Part model, mm, in its own coordinate system. A direction names the side the tool comes from. Give positions to 0.01 mm unless a question says otherwise; leave off trailing zeros. Write each loop counter-clockwise with the first axis right and the second up, starting at its lowest first coordinate (ties: lowest second). Pieces come first, ordered by that corner, then holes.
Autodesk Inventor part; units mm, degrees
ref_plane "YZ Plane" through (0, 0, 0) normal (1, 0, 0) x (0, 1, 0)
ref_plane "XZ Plane" through (0, 0, 0) normal (0, 1, 0) x (-1, 0, 0)
ref_plane "XY Plane" through (0, 0, 0) normal (0, 0, 1) x (1, 0, 0)
sketch "Sketch1" plane through (0, 0, 0) normal (0, 0, 1) x (1, 0, 0)
  line L0 (-25.4, 15.875) -> (-25.4, 3.175)
  line L1 (-25.4, 3.175) -> (9.525, 3.175)
  line L2 (9.525, 3.175) -> (9.525, 15.875)
  line L3 (9.525, 15.875) -> (-25.4, 15.875)
  dimension "d0" = 12.7
  dimension "d1" = 34.925
extrude "Extrusion1" add sketch "Sketch1" along normal blind 4.7625
hole "Hole1" at (3.175, 9.525, 4.7625) direction (0, 0, -1) diameter 4.318 end through all countersink diameter 8.4328 countersink angle 82
hole "Hole2" at (-9.525, 9.525, 4.7625) direction (0, 0, -1) diameter 3.302 end through all
sketch "Sketch2" plane through (0, 0, 4.7625) normal (0, 0, 1) x (1, 0, 0)
  line L0 (-25.4, 15.875) -> (9.525, 15.875)
  line L1 (-25.4, 3.175) -> (-25.4, 15.875)
  line L2 (-25.4, 11.1125) -> (-22.225, 11.1125)
  line L3 (-22.225, 11.1125) -> (-22.225, 7.9375)
  line L4 (-22.225, 7.9375) -> (-25.4, 7.9375)
  line L5 (-25.4, 7.9375) -> (-25.4, 11.1125)
  arc A0 (-22.225, 7.9375) -> (-22.225, 11.1125) centre (-22.225, 9.525) ccw
  dimension "d22" = 3.175
  dimension "d23" = 6.35
  dimension "d24" = 3.175
extrude "Extrusion2" cut sketch "Sketch2" against normal blind 1.016 contours L1 L2 L3 L4
sketch "Sketch6" plane through (-25.4, 3.175, 0) normal (0, -1, 0) x (1, 0, 0)
  line L0 (0, 0) -> (0, 4.7625)
  line L1 (0, 0) -> (34.925, 0)
  line L2 (0, 2.3813) -> (12.7, 0)
  line L3 (0, 0) -> (12.7, 0)
  line L4 (0, 0) -> (0, 2.3813)
  line L5 (0, 0) -> (12.7, 0)
  dimension "d35" = 2.3813
  dimension "d132" = 12.7
extrude "Extrusion5" cut sketch "Sketch6" against normal through all
hole "Hole4" at (-15.875, 13.4938, 4.7625) direction (0, 0, -1) diameter 0.7874 end through all
hole "Hole6" at (-15.875, 5.5563, 4.7625) direction (0, 0, -1) diameter 0.7874 end through all
sketch "Sketch8" plane through (0, 0, 4.7625) normal (0, 0, 1) x (1, 0, 0)
  line L0 (-25.4, 11.1125) -> (-22.225, 11.1125)
  line L1 (-22.225, 11.1125) -> (-22.225, 7.9375)
  line L2 (-25.4, 11.1125) -> (-22.225, 11.1125)
  line L3 (-22.225, 10.3187) -> (-25.4, 11.1125)
  line L4 (-22.225, 11.1125) -> (-22.225, 10.3187)
  line L5 (-22.225, 8.7312) -> (-25.4, 7.9375)
  line L6 (-22.225, 7.9375) -> (-22.225, 8.7312)
  dimension "d80" = 0.7937
  dimension "d81" = 0.7937
extrude "Extrusion7" add sketch "Sketch8" against normal up to next
sketch "Sketch10" plane through (0, 0, 4.7625) normal (0, 0, 1) x (1, 0, 0)
  line L0 (-22.225, 10.3187) -> (-22.225, 7.9375)
  line L1 (-22.225, 7.9375) -> (-25.4, 7.9375)
  line L2 (-22.225, 8.7312) -> (-25.4, 7.9375)
  line L3 (-22.225, 7.9375) -> (-22.225, 8.7312)
  dimension "d85" = 0.7937
extrude "Extrusion8" add sketch "Sketch10" against normal up to next
sketch "Sketch12" plane through (0, 0, 4.7625) normal (0, 0, 1) x (1, 0, 0)
  line L0 (-25.4, 15.875) -> (9.525, 15.875)
  line L1 (-25.4, 11.1125) -> (-25.4, 15.875)
  line L2 (-22.225, 10.3187) -> (-22.225, 8.7312)
  line L3 (-25.4, 11.9062) -> (-12.7, 15.875)
  line L4 (-25.4, 15.875) -> (-25.4, 11.9062)
  dimension "d88" = 12.7
  dimension "d89" = 3.9688
extrude "Extrusion9" cut sketch "Sketch12" against normal through all
sketch "Sketch13" plane through (0, 0, 4.7625) normal (0, 0, 1) x (1, 0, 0)
  line L0 (-25.4, 3.175) -> (-25.4, 7.9375)
  line L1 (9.525, 3.175) -> (-25.4, 3.175)
  line L2 (-12.7, 15.875) -> (9.525, 15.875)
  line L3 (-12.7, 3.175) -> (-25.4, 3.175)
  line L4 (-25.4, 7.1437) -> (-12.7, 3.175)
  dimension "d92" = 12.7
  dimension "d93" = 3.9688
extrude "Extrusion10" cut sketch "Sketch13" against normal through all
hole "Hole7" at (-0.7937, 13.4938, 4.7625) direction (0, 0, -1) diameter 2.159 end through all
hole "Hole8" at (-0.7937, 5.5562, 4.7625) direction (0, 0, -1) diameter 2.159 end through all
hole "Hole9" at (7.1437, 13.4938, 4.7625) direction (0, 0, -1) diameter 2.159 end through all
hole "Hole10" at (7.1437, 5.5562, 4.7625) direction (0, 0, -1) diameter 2.159 end through all
sketch "Sketch14" plane through (0, 0, 4.7625) normal (0, 0, 1) x (1, 0, 0)
  line L0 (-25.4, 11.1125) -> (-22.225, 10.3187)
  line L1 (-22.225, 8.7312) -> (-25.4, 7.9375)
  arc A0 (-22.225, 8.7312) -> (-22.225, 10.3187) centre (-22.4234, 9.525) ccw
  line L2 (-22.225, 10.3187) -> (-22.225, 8.7312)
  line L3 (-22.225, 8.7312) -> (-22.225, 10.3187)
  point P0 (0, 0)
extrude "Extrusion11" cut sketch "Sketch14" against normal up to surface (1.016 mm away)
properties part number "J005774" material "STAINLESS STEEL, 303"
1) Mould opens along X. For faces 3 (the flat face through (-2, 10, 0)), 4 (the cylindrical face through (8.101, 5.058, 2.348)), 5 (the cylindrical face through (-0.38, 4.56, 2.35)), 6 (the cylindrical face through (-21.605, 9.51, 4.262)) say: +X half, -X half, draft (parallel to the pull), parting line (faces both ways), or undercut.
Check result:
face 3: draft
face 4: undercut
face 5: undercut
face 6: -X half
2) 3-axis set-ups, long thin cutter, end or side, ignore diameter. For faces 1 (the conical face through (5.44, 9.82, 2.54)), 2 (the flat face through (-23.79, 10.71, 4.26)): which of +Z, -Z, +X, -X, +Y, -Y reach the whole face in a straight line?
Check result:
face 1: +Z
face 2: +Z, -X
3) Saw through at A-A (z = 1). State how many separate pieces and enclosed holes the cut face has, and give its area (3 significant figures).
Check result:
separate pieces: 1
enclosed holes: 8
area: 302 mm2
4) Drill centre lines: L1, parallel to Y at x = -10, z = 4.1 (3 decimals); L2, parallel to Y at x = -0.5, z = 1.65 (3 decimals); L3, parallel to Y at x = 5, z = 3.4 (3 decimals). Where is each one in solid material? Low to high.
Check result:
L1: y = 3.175 to 7.944, 11.106 to 15.875
L2: y = 3.175 to 4.517, 6.595 to 12.455, 14.533 to 15.875
L3: y = 3.175 to 7.104, 11.946 to 15.875
5) Flat gauge pins, fed straight in: P1, Ø3, axis at x = -15.5, y = 9.5, coming from the -Z side; P2, Ø1.6, axis at x = -23, y = 9.5, coming from the +Z side. Where does each tip first touch, or does it go through?
Check result:
P1: stops at z = 0.24
P2: stops at z = 3.75
6) Saw through at B-B (x = -14). Write the cut outline in (y, z).
Check result:
outline: (3.58, 0.24) - (15.47, 0.24) - (15.47, 4.76) - (3.58, 4.76) - close
